Part model, mm, in its own coordinate system. A direction names the side the tool comes from. Round coordinates to 2 decimals unless told otherwise and drop trailing zeros. Loops run counter-clockwise (first coordinate to the right, second up) from the corner with the lowest first, then second, coordinate; pieces in that order, holes last. Notation, with made-up numbers: (-24, 22.5) -> (8, 22.5) arc R20 cw to (8, 51.5) -> close; hole circle Ø3 at (11.5, 78.25). An arc over 180 degrees is marked (long way). Use a Markdown table: item, result. Add a question column.
Item 1: Flat gauge pins, fed straight in: pin 1 (1 mm diameter, centred on x = 25.5, z = -42, fed in from -Y); pin 2 (2.5 mm diameter, centred on x = 26.5, y = -6, fed in from +Z); pin 3 (2.5 mm diameter, centred on y = -5.5, z = -44, fed in from -X). Where does each tip first touch, or does it go through?
Item 2: Cut at C-C, the plane y = -5. List the corners of the cut face in (x, z), plus the area to 3 significant figures.
Item 3: Probe line 1 (X direction, y = -4.75, z = -15); line 2 (Z direction, x = 19, y = -3.75); line 3 (Y direction, x = 7, z = -14). List the from-to ranges inside material, lowest first. Write a range as [from, to].
Item 4: Two-plate mould, pull along Z, no slides. Class faces 1 (the face through (44, -6, -3)), 2 (the face through (23, 0, -51)), 3 (the face through (24, -5, -3.5)): pulls with the +Z half, pulls with the -Z half, needs draft (parallel to the pull), parting line crosses it, or undercut.
Item 5: Which spindle directions (+Z, -Z, +X, -X, +Y, -Y) get a long thin tool onto all of the face, cutting with end or side? Do faces 4 (the face through (3.5, -5, -45)), 5 (the face through (44.5, -6, -47)), 6 (the face through (2, -6, -47)), 7 (the face through (23, -6, -2)). Say none if no direction does.
Item 6: Cut at A-A, the plane x = 23.5. List the corners of the cut face in (y, z), plus the area to 3 significant figures.
Item 7: Cut at B-B, the plane z = -65.5. List the corners of the cut face in (x, y), plus the area to 3 significant figures.
```python
from build123d import *

# Parameters (mm, degrees)
EXTRUDE_1_DEPTH     = 4
CUT_EXTRUDE_1_DEPTH = 1.5
EXTRUDE_START       = 3
EXTRUDE_2_DEPTH     = 3
CHAMFER_1_SIZE      = 3
FILLET_1_R          = 3


with BuildPart() as part:
    # Эскиз1 → Бобышка-Вытянуть1 (new body)
    with BuildSketch(Plane(origin=(0, 0, 0), x_dir=(1, 0, 0), z_dir=(0, 1, 0))):
        with BuildLine():
            Line((4.5, 0), (42, 0))
            ThreePointArc((42, 0), (45.181980515, 1.318019485), (46.5, 4.5))
            Line((46.5, 4.5), (46.5, 87))
            ThreePointArc((46.5, 87), (42.692388155, 96.192388155), (33.5, 100))
            Line((33.5, 100), (13, 100))
            ThreePointArc((13, 100), (3.807611845, 96.192388155), (0, 87))
            Line((0, 87), (0, 4.5))
            ThreePointArc((0, 4.5), (1.318019485, 1.318019485), (4.5, 0))
        make_face()
    extrude(amount=-EXTRUDE_1_DEPTH)

    # Эскиз2 → Вырез-Вытянуть1 (cut)
    with BuildSketch(Plane.XZ.offset(4)):
        with BuildLine():
            Line((3.5, -4.5), (3.5, -87))
            ThreePointArc((3.5, -87), (6.282485579, -93.717514421), (13, -96.5))
            Line((13, -96.5), (33.5, -96.5))
            ThreePointArc((33.5, -96.5), (40.217514421, -93.717514421), (43, -87))
            Line((43, -87), (43, -4.5))
            ThreePointArc((43, -4.5), (42.707106781, -3.792893219), (42, -3.5))
            Line((42, -3.5), (4.5, -3.5))
            ThreePointArc((4.5, -3.5), (3.792893219, -3.792893219), (3.5, -4.5))
        make_face()
    extrude(amount=-CUT_EXTRUDE_1_DEPTH, mode=Mode.SUBTRACT)

    # Эскиз3 → Бобышка-Вытянуть2 (add)
    with BuildSketch(Plane(origin=(0, -4, 0), x_dir=(-1, 0, 0), z_dir=(0, -1, 0)).offset(EXTRUDE_START)):
        with BuildLine():
            Line((-2, 87), (-2, 4.5))
            ThreePointArc((-2, 4.5), (-2.732233047, 2.732233047), (-4.5, 2))
            Line((-4.5, 2), (-42, 2))
            ThreePointArc((-42, 2), (-43.767766953, 2.732233047), (-44.5, 4.5))
            Line((-44.5, 4.5), (-44.5, 87))
            Line((-44.5, 87), (-43, 87))
            Line((-43, 87), (-43, 4.5))
            ThreePointArc((-43, 4.5), (-42.707106781, 3.792893219), (-42, 3.5))
            Line((-42, 3.5), (-4.5, 3.5))
            ThreePointArc((-4.5, 3.5), (-3.792893219, 3.792893219), (-3.5, 4.5))
            Line((-3.5, 4.5), (-3.5, 87))
            Line((-3.5, 87), (-2, 87))
        make_face()
    extrude(amount=-EXTRUDE_2_DEPTH)

    # Фаска1
    # the kernel refuses this chamfer: 3 mm, written as the material it adds along each edge
    with BuildSketch(Plane(origin=(11.215048964, -4, -87), x_dir=(0, 0.027495876610586334, -0.9996219169112968), z_dir=(-1, 0, 0))) as chamfer_1_piece_1_section:
        Polygon((CHAMFER_1_SIZE * 0.999621916911, CHAMFER_1_SIZE * 0.0274958766106), (-CHAMFER_1_SIZE * 0.0274958766106, CHAMFER_1_SIZE * 0.999621916911), (0, 0), align=None)
    chamfer_1_piece_1 = extrude(amount=9.215048964, mode=Mode.PRIVATE)
    chamfer_1_piece_1 = chamfer_1_piece_1 - Plane(origin=(13, -4.5189099, -87), x_dir=(-1, 0, 0), z_dir=(0, -1, 0)) * Cylinder(9.5, 31, mode=Mode.PRIVATE)
    chamfer_1_piece_1 = split(chamfer_1_piece_1, bisect_by=Plane(origin=(3.605353411, -7, -88.883676774), z_dir=(0, 1, 0)), keep=Keep.TOP, mode=Mode.PRIVATE)
    add(chamfer_1_piece_1)
    with BuildSketch(Plane(origin=(44.5, -4, -87), x_dir=(0, 0.027495876610586334, -0.9996219169112968), z_dir=(-1, 0, 0))) as chamfer_1_piece_2_section:
        Polygon((CHAMFER_1_SIZE * 0.999621916911, CHAMFER_1_SIZE * 0.0274958766106), (-CHAMFER_1_SIZE * 0.0274958766106, CHAMFER_1_SIZE * 0.999621916911), (0, 0), align=None)
    chamfer_1_piece_2 = extrude(amount=9.215048964, mode=Mode.PRIVATE)
    chamfer_1_piece_2 = chamfer_1_piece_2 - Plane(origin=(33.5, -4.985903001, -87), x_dir=(0, 0, -1), z_dir=(0, -1, 0)) * Cylinder(9.5, 31, mode=Mode.PRIVATE)
    chamfer_1_piece_2 = split(chamfer_1_piece_2, bisect_by=Plane(origin=(43.75, -7, -87.991212463), z_dir=(0, 1, 0)), keep=Keep.TOP, mode=Mode.PRIVATE)
    add(chamfer_1_piece_2)

    # Скругление1
    fillet_1_edges = [part.edges().sort_by_distance(p)[0] for p in [
        (23.25, 0, 0),
        (1.318019485, 0, -1.318019485),
        (0, 0, -45.75),
        (3.807611845, 0, -96.192388155),
        (23.25, 0, -100),
        (42.692388155, 0, -96.192388155),
        (46.5, 0, -45.75),
        (45.181980515, 0, -1.318019485),
    ]]
    fillet(fillet_1_edges, radius=FILLET_1_R)


solid = part.part
```
A:
| question | item | result |
|---|---|---|
| 1 | pin 1 | stops at y = -2.5 |
| 1 | pin 2 | stops at z = -2 |
| 1 | pin 3 | stops at x = 2 |
| 2 | outline | (2, -89) -> (3.71, -89) arc R9.5 cw to (3.5, -87) -> (3.5, -4.5) arc R1 cw to (4.5, -3.5) -> (42, -3.5) arc R1 cw to (43, -4.5) -> (43, -87) arc R9.5 cw to (42.79, -89) -> (44.5, -89) -> (44.5, -4.5) arc R2.5 ccw to (42, -2) -> (4.5, -2) arc R2.5 ccw to (2, -4.5) -> close |
| 2 | area | 318 mm^2 |
| 3 | line 1 | x = [2, 3.5], [43, 44.5] |
| 3 | line 2 | z = [-100, -96.5], [-3.5, 0] |
| 3 | line 3 | y = [-2.5, 0] |
| 4 | face 1 | pulls with the +Z half |
| 4 | face 2 | needs draft |
| 4 | face 3 | undercut |
| 5 | face 4 | -Y |
| 5 | face 5 | +Z, -Z, +X, -Y |
| 5 | face 6 | +Z, -Z, -X, -Y |
| 5 | face 7 | +Z, +X, -X, -Y |
| 6 | outline | (-7, -3.5) -> (-2.5, -3.5) -> (-2.5, -96.5) -> (-4, -96.5) -> (-4, -100) -> (-3, -100) arc R3 ccw to (0, -97) -> (0, -3) arc R3 ccw to (-3, 0) -> (-4, 0) -> (-4, -2) -> (-7, -2) -> close |
| 6 | area | 261 mm^2 |
| 7 | outline | (0, -4) -> (2, -4) -> (2, -7) -> (3.5, -7) -> (3.5, -2.5) -> (43, -2.5) -> (43, -7) -> (44.5, -7) -> (44.5, -4) -> (46.5, -4) -> (46.5, -3) arc R3 ccw to (43.5, 0) -> (3, 0) arc R3 ccw to (0, -3) -> close |
| 7 | area | 132 mm^2 |
